For this review, take the finished solid that the model builds, in its own axes (mm). A direction names the side the tool comes from. Give positions to 0.01 mm unless a question says otherwise; leave off trailing zeros. Write each loop counter-clockwise with the first axis right and the second up, starting at its lowest first coordinate (ties: lowest second). Pieces come first, ordered by that corner, then holes.
Q1. We need section D-D (x = 13). Write out the cut boundary in (y, z).
Q2. For line 1 (Y direction, x = 0, z = 87.85); line 2 (Y direction, x = 0, z = 50); line 3 (Z direction, x = 9.5, y = 18), list the stretches that pass through material, from the lowest coordinate up.
Q3. We need section B-B (z = 3). Write out the cut boundary in (x, y).
Q4. Insertion check: P1, Ø5, axis at x = -5, z = 35, coming from the +Y side; P2, Ø11.5, axis at x = 0, y = 0, coming from the -Z side; P3, Ø3, axis at x = 10.5, z = 36.5, coming from the -Y side; P4, Ø10.5, axis at x = 16.5, y = -16.5, coming from the -Z side. Each pin has a flat end and moves straight along its axis. Give the tip position at first contact, or say it passes through.
Q5. Mouldability with a two-part tool opening along Y and no side actions: class faces 1 (the cylindrical face through (5.158, -3.955, 39.384)), 2 (the flat face through (-20, 0, 39)), 3 (the cylindrical face through (-19.443, -11.323, 81.73)), 4 (the flat face through (0, -20, 39)) as released by +Y, released by -Y, zero draft, split by the parting line, or undercut.
Q6. Machinability: for faces 5 (the flat face through (21, 0, 0)), 6 (the flat face through (0, 21, 0)), 7 (the flat face through (17, -17, 80)), 8 (the flat face through (-4, 6, 84)), which of the approach directions +Z, -Z, +X, -X, +Y, -Y give a long, thin tool a straight path to every point of the face, cutting with its end or side? Answer none if there is none.
```python
from build123d import *

# Parameters (mm, degrees)
EXTRUDE_1_DEPTH     = 80
SKETCH_3_R          = 22.5
EXTRUDE_2_DEPTH     = 10
EXTRUDE_START       = 10
SKETCH_4_R          = 22.5
EXTRUDE_3_DEPTH     = 10
SKETCH_6_R          = 9.5
CUT_EXTRUDE_3_DEPTH = 6
CUT_EXTRUDE_START   = -6
SKETCH_7_R          = 9.5
CUT_EXTRUDE_4_DEPTH = 6
SKETCH_8_R          = 6.5
CUT_EXTRUDE_5_DEPTH = 100
CUT_EXTRUDE_START_2 = -6.49
SKETCH_9_R          = 22.5
SKETCH_9_R_2        = 19.5
CUT_EXTRUDE_7_DEPTH = 3.1


with BuildPart() as part:
    # 草图1 → 凸台-拉伸1 (new body)
    with BuildSketch(Plane.XY):
        Polygon((-20, 18), (-18, 20), (17.735809733, 20), (20, 18), (20, -17.735809733), (17.735809733, -20), (-18, -20), (-20, -18), align=None)
    extrude(amount=EXTRUDE_1_DEPTH)

    # 草图3 → 凸台-拉伸2 (add)
    with BuildSketch(Plane.XY.offset(80)):
        with Locations(Location((0, 0, 0), (0, 0, 152.733955549))):
            Circle(SKETCH_3_R)
    extrude(amount=EXTRUDE_2_DEPTH)

    # 草图4 → 凸台-拉伸3 (add)
    with BuildSketch(Plane(origin=(0, 0, 0), x_dir=(-1, 0, 0), z_dir=(0, 0, -1)).offset(EXTRUDE_START)):
        with Locations(Location((0, 0, 0), (0, 0, 27.266044451))):
            Circle(SKETCH_4_R)
    extrude(amount=-EXTRUDE_3_DEPTH)

    # 草图6 → 切除-拉伸3 (cut)
    with BuildSketch(Plane(origin=(0, 0, -10), x_dir=(-1, 0, 0), z_dir=(0, 0, -1))):
        Circle(SKETCH_6_R)
    extrude(amount=-CUT_EXTRUDE_3_DEPTH, mode=Mode.SUBTRACT)

    # 草图7 → 切除-拉伸4 (cut)
    with BuildSketch(Plane.XY.offset(90).offset(CUT_EXTRUDE_START)):
        with Locations(Location((0, 0, 0), (0, 0, 180))):
            Circle(SKETCH_7_R)
    extrude(amount=CUT_EXTRUDE_4_DEPTH, mode=Mode.SUBTRACT)

    # 草图8 → 切除-拉伸5 (cut)
    with BuildSketch(Plane(origin=(0, 0, -10), x_dir=(-1, 0, 0), z_dir=(0, 0, -1))):
        Circle(SKETCH_8_R)
    extrude(amount=-CUT_EXTRUDE_5_DEPTH, mode=Mode.SUBTRACT)

    # 草图9 → 切除-拉伸7 (cut)
    with BuildSketch(Plane.XY.offset(90).offset(CUT_EXTRUDE_START_2)):
        with Locations(Location((0, 0, 0), (0, 0, 152.733955549))):
            Circle(SKETCH_9_R)
        Circle(SKETCH_9_R_2, mode=Mode.SUBTRACT)
    extrude(amount=CUT_EXTRUDE_7_DEPTH, mode=Mode.SUBTRACT)


solid = part.part
```
Computed:
1. outline: (-20, 0) - (-18.36, 0) - (-18.36, -10) - (18.36, -10) - (18.36, 0) - (20, 0) - (20, 80) - (18.36, 80) - (18.36, 83.51) - (14.53, 83.51) - (14.53, 86.61) - (18.36, 86.61) - (18.36, 90) - (-18.36, 90) - (-18.36, 86.61) - (-14.53, 86.61) - (-14.53, 83.51) - (-18.36, 83.51) - (-18.36, 80) - (-20, 80) - close
2. line 1: y = -22.5 to -9.5, 9.5 to 22.5
2. line 2: y = -20 to -6.5, 6.5 to 20
2. line 3: z = -10 to 83.51, 86.61 to 90
3. outline: (-20, -18) - (-18, -20) - (17.74, -20) - (20, -17.74) - (20, 18) - (17.74, 20) - (-18, 20) - (-20, 18) - close; hole circle Ø13 at (0, 0)
4. P1: stops at y = 20
4. P2: passes through
4. P3: stops at y = -20
4. P4: stops at z = -10
5. face 1: undercut
5. face 2: zero draft
5. face 3: split by the parting line
5. face 4: released by -Y
6. face 5: +X, +Y, -Y
6. face 6: +X, -X, +Y
6. face 7: +Z, +X, -Y
6. face 8: +Z
